Check sheet for the drawn part. Datum: minimum x, y, z corner. Units: mm. A direction names the side the tool comes from. Coordinates: 2 decimals unless noted, no trailing zeros. Put each result on its own line as item: value.
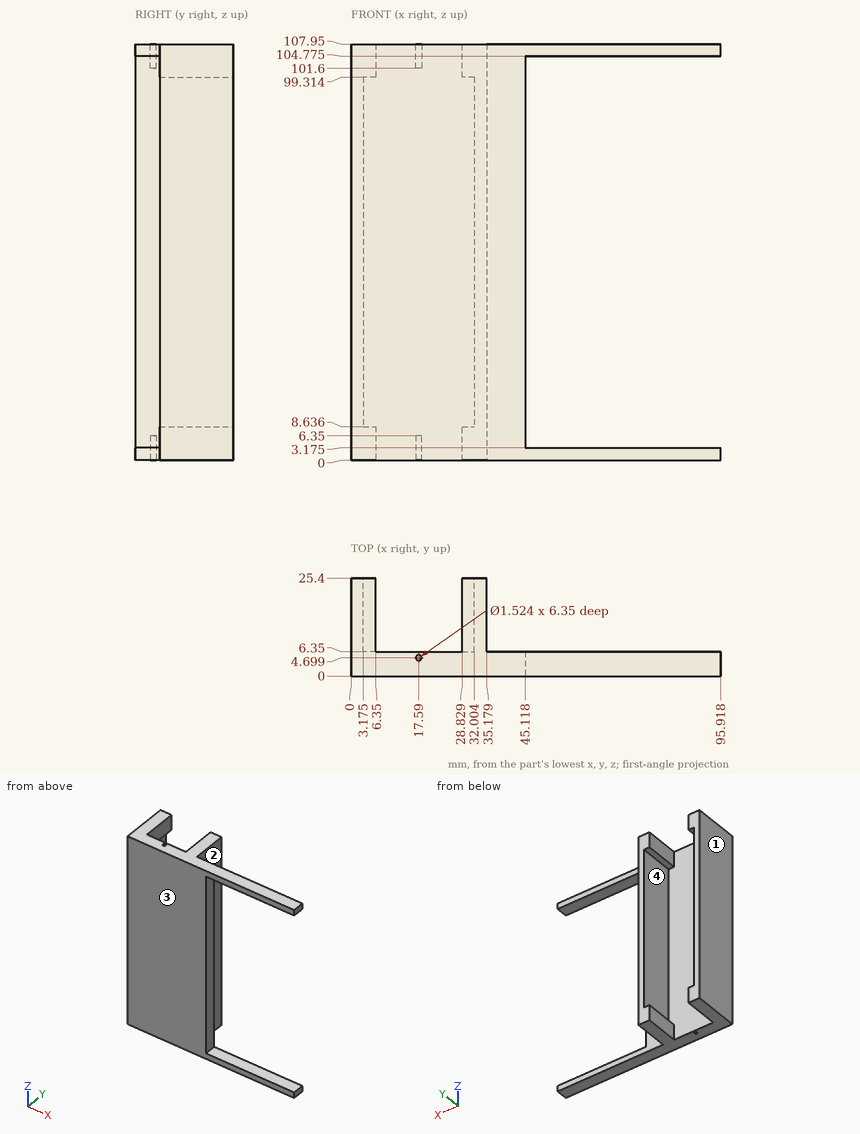
Q1. Access from +Z, -Z, +X, -X, +Y, -Y to the whole of each face (thin tool, end or side, straight path). Record for the marked faces 1 and 2.
Answer block:
face 1: +Z, -Z, -X, +Y, -Y
face 2: +Z, -Z, +X, +Y
Q2. Draft check along Z on the marked faces 3 and 4. Enter one of: pulls with the +Z half, pulls with the -Z half, needs draft (parallel to the pull), parting line crosses it, or undercut.
Answer block:
face 3: needs draft
face 4: undercut
Q3. Thickness scan on L1, parallel to X at y = 11, z = 28 (1 decimal); L2, parallel to X at y = 21.75, z = 100.5; L3, parallel to Y at x = 38.5, z = 84. Record the ranges inside material, lowest first. Write a range as [from, to].
Answer block:
L1: x = [0, 3.2], [32, 35.2]
L2: x = [0, 6.35], [28.83, 35.18]
L3: y = [0, 6.35]
Q4. Depth check by flat-ended pin: pin 1 Ø4.5 at (y, z) = (17.5, 4.5) entering from +X; pin 2 Ø1.9 at (y, z) = (2.5, 34.5) entering from +X. Enter the tip coordinate at first touch or a pass-through.
Answer block:
pin 1: stops at x = 35.18
pin 2: stops at x = 45.12
